Design review of the part built by this model. Coordinates are the model's own, in mm. Face numbers are marked on the shaded views. A direction names the side the tool comes from. Coordinates: 2 decimals unless noted, no trailing zeros. Loops run counter-clockwise (first coordinate to the right, second up) from the corner with the lowest first, then second, coordinate; pieces in that order, holes last. Notation, with made-up numbers: M 77,77.5 L 126,77.5 A19 ccw 126,93.5 Z; hole C 71,-25.75 d10. An arc over 180 degrees is marked long. Put each result on its own line as item: value. Start each with the question number.
(1) Take a section at D-D, the plane x = 66. Give the boundary of the cut face in (y, z).
(2) For probe 1 along Y at (x, z) = (12.7, 11); probe 2 along Y at (x, z) = (50.8, 14.5); probe 3 along Z at (x, y) = (93.5, 104), list the stretches that pass through material, from the lowest coordinate up. Write a range as [from, to].
(3) For the marked faces 1 and 2, list the 3-axis set-ups (+Z, -Z, +X, -X, +Y, -Y) from which the entire face can be reached by the end or side of a thin tool; tool diameter is ignored.
(4) Take a section at A-A, the plane y = 114.3. Give the boundary of the cut face in (x, z).
(5) Take a section at B-B, the plane x = 88.9. Give the boundary of the cut face in (y, z).
(6) Take a section at C-C, the plane z = 16. Give the boundary of the cut face in (x, y).
(7) The part is to be moulded in two halves that separate along X. For the marked faces 3, 4, 5 and 6, say which applies: +X half, -X half, draft (parallel to the pull), parting line (faces both ways), or undercut.
(8) Clearance check with flat-ended pins moving along their axes: pin 1 (3 mm diameter, centred on x = 62, z = 3, fed in from -Y); pin 2 (11.5 mm diameter, centred on x = 12.7, y = 25.4, fed in from -Z); pin 3 (1.9 mm diameter, centred on x = 54, z = 3.5, fed in from +Y); pin 4 (10 mm diameter, centred on x = 16, y = 29.5, fed in from -Z). State where each tip first meets the part, or that it passes through.
```python
from build123d import *

# Parameters (mm, degrees)
SKETCH1_W           = 101.6
SKETCH1_H           = 127
BOSS_EXTRUDE1_DEPTH = 19.05
SKETCH2_W           = 25.4
SKETCH2_H           = 127
CUT_EXTRUDE1_DEPTH  = 6.35
CUT_EXTRUDE2_REACH  = 165.751
SKETCH4_R           = 6.35
SKETCH9_W           = 50.8
SKETCH9_H           = 50.8
CUT_EXTRUDE7_DEPTH  = 6.35
SKETCH11_R          = 6.35
CUT_EXTRUDE8_DEPTH  = 9.525


with BuildPart() as part:
    # Sketch1 → Boss-Extrude1 (new body)
    with BuildSketch(Plane.XY):
        with Locations((50.8, 63.5)):
            Rectangle(SKETCH1_W, SKETCH1_H)
    extrude(amount=BOSS_EXTRUDE1_DEPTH)

    # Sketch2 → Cut-Extrude1 (cut)
    with BuildSketch(Plane(origin=(0, 0, 0), x_dir=(-1, 0, 0), z_dir=(0, 0, -1))):
        with Locations((-88.9, 63.5)):
            Rectangle(SKETCH2_W, SKETCH2_H)
        with Locations((-12.7, 63.5)):
            Rectangle(SKETCH2_W, SKETCH2_H)
    extrude(amount=-CUT_EXTRUDE1_DEPTH, mode=Mode.SUBTRACT)

    # Sketch4 → Cut-Extrude2 (cut, up to next)
    with BuildSketch(Plane.XY.offset(19.05), mode=Mode.PRIVATE) as cut_extrude2_sk1:
        with Locations((12.7, 114.3)):
            Circle(SKETCH4_R)
    cut_extrude2_tool1 = extrude(cut_extrude2_sk1.sketch, amount=-CUT_EXTRUDE2_REACH, mode=Mode.PRIVATE) & part.part
    # Sketch4 → Cut-Extrude2 (cut, up to next)
    with BuildSketch(Plane.XY.offset(19.05), mode=Mode.PRIVATE) as cut_extrude2_sk2:
        with Locations((12.7, 25.4)):
            Circle(SKETCH4_R)
    cut_extrude2_tool2 = extrude(cut_extrude2_sk2.sketch, amount=-CUT_EXTRUDE2_REACH, mode=Mode.PRIVATE) & part.part
    # Sketch4 → Cut-Extrude2 (cut, up to next)
    with BuildSketch(Plane.XY.offset(19.05), mode=Mode.PRIVATE) as cut_extrude2_sk3:
        with Locations(Location((88.9, 25.4, 0), (0, 0, 180))):
            Circle(SKETCH4_R)
    cut_extrude2_tool3 = extrude(cut_extrude2_sk3.sketch, amount=-CUT_EXTRUDE2_REACH, mode=Mode.PRIVATE) & part.part
    # Sketch4 → Cut-Extrude2 (cut, up to next)
    with BuildSketch(Plane.XY.offset(19.05), mode=Mode.PRIVATE) as cut_extrude2_sk4:
        with Locations(Location((88.9, 114.3, 0), (0, 0, 180))):
            Circle(SKETCH4_R)
    cut_extrude2_tool4 = extrude(cut_extrude2_sk4.sketch, amount=-CUT_EXTRUDE2_REACH, mode=Mode.PRIVATE) & part.part
    add(cut_extrude2_tool1.solids().sort_by_distance((12.7, 114.3, 19.05))[0], mode=Mode.SUBTRACT)
    add(cut_extrude2_tool2.solids().sort_by_distance((12.7, 25.4, 19.05))[0], mode=Mode.SUBTRACT)
    add(cut_extrude2_tool3.solids().sort_by_distance((88.9, 25.4, 19.05))[0], mode=Mode.SUBTRACT)
    add(cut_extrude2_tool4.solids().sort_by_distance((88.9, 114.3, 19.05))[0], mode=Mode.SUBTRACT)

    # Sketch9 → Cut-Extrude7 (cut)
    with BuildSketch(Plane(origin=(0, 0, 0), x_dir=(-1, 0, 0), z_dir=(0, 0, -1))):
        with Locations((-50.8, 25.4)):
            Rectangle(SKETCH9_W, SKETCH9_H)
        with Locations((-50.8, 101.6)):
            Rectangle(SKETCH9_W, SKETCH9_H)
    extrude(amount=-CUT_EXTRUDE7_DEPTH, mode=Mode.SUBTRACT)

    # Sketch11 → Cut-Extrude8 (cut)
    with BuildSketch(Plane.XY.offset(19.05)):
        with Locations((50.8, 63.5)):
            Circle(SKETCH11_R)
    extrude(amount=-CUT_EXTRUDE8_DEPTH, mode=Mode.SUBTRACT)


solid = part.part
```
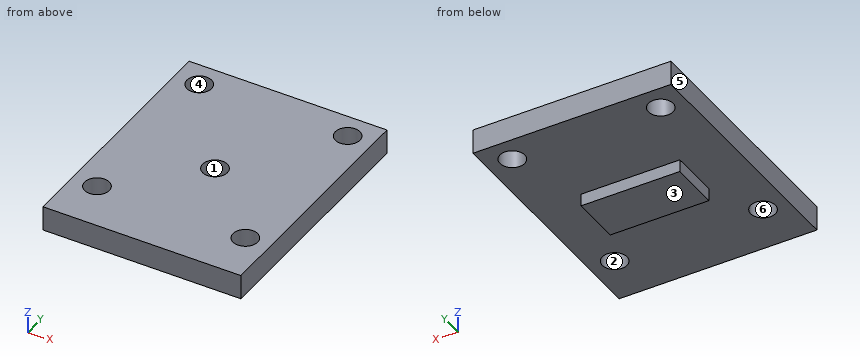
Computed values:
1. outline: M 0,6.35 L 50.8,6.35 L 50.8,0 L 76.2,0 L 76.2,6.35 L 127,6.35 L 127,19.05 L 0,19.05 Z
2. probe 1: y = [0, 19.05], [31.75, 107.95], [120.65, 127]
2. probe 2: y = [0, 57.15], [69.85, 127]
2. probe 3: z = [6.35, 19.05]
3. face 1: +Z
3. face 2: +Z, -Z
4. outline: M 0,6.35 L 6.35,6.35 L 6.35,19.05 L 0,19.05 Z; M 19.05,6.35 L 82.55,6.35 L 82.55,19.05 L 19.05,19.05 Z; M 95.25,6.35 L 101.6,6.35 L 101.6,19.05 L 95.25,19.05 Z
5. outline: M 0,6.35 L 19.05,6.35 L 19.05,19.05 L 0,19.05 Z; M 31.75,6.35 L 107.95,6.35 L 107.95,19.05 L 31.75,19.05 Z; M 120.65,6.35 L 127,6.35 L 127,19.05 L 120.65,19.05 Z
6. outline: M 0,0 L 101.6,0 L 101.6,127 L 0,127 Z; hole C 12.7,25.4 d12.7; hole C 12.7,114.3 d12.7; hole C 50.8,63.5 d12.7; hole C 88.9,25.4 d12.7; hole C 88.9,114.3 d12.7
7. face 3: draft
7. face 4: undercut
7. face 5: -X half
7. face 6: undercut
8. pin 1: stops at y = 50.8
8. pin 2: passes through
8. pin 3: stops at y = 76.2
8. pin 4: stops at z = 6.35
